Source: CAD feature listing. Evaluate the final solid. Frame: model axes, mm. A direction names the side the tool comes from. Give positions to 0.01 mm unless a question says otherwise; leave off trailing zeros. Loops run counter-clockwise (first coordinate to the right, second up) from the corner with the lowest first, then second, coordinate; pieces in that order, holes last.
from build123d import *

# Parameters (mm, degrees)
SKETCH2_R           = 3.25
SKETCH2_R_2         = 5.25
SKETCH2_R_3         = 2.5
BOSS_EXTRUDE1_DEPTH = 2.5


with BuildPart() as part:
    # Sketch2 → Boss-Extrude1 (new, symmetric)
    with BuildSketch(Plane.XY):
        with BuildLine():
            Line((0, 40), (0, 10))
            ThreePointArc((0, 10), (8.556304179, 0.104761631), (19.583148475, 7.142857143))
            ThreePointArc((19.583148475, 7.142857143), (21.025950646, 9.207134903), (23.416407865, 10))
            Line((23.416407865, 10), (66.583592135, 10))
            ThreePointArc((66.583592135, 10), (68.974049354, 9.207134903), (70.416851525, 7.142857143))
            ThreePointArc((70.416851525, 7.142857143), (81.443695821, 0.104761631), (90, 10))
            Line((90, 10), (90, 20))
            ThreePointArc((90, 20), (88.828427125, 22.828427125), (86, 24))
            Line((86, 24), (70, 24))
            ThreePointArc((70, 24), (50.388386486, 28.00668945), (33.919878771, 39.384615385))
            ThreePointArc((33.919878771, 39.384615385), (33.261138462, 39.839732422), (32.476673921, 40))
            Line((32.476673921, 40), (23.416407865, 40))
            ThreePointArc((23.416407865, 40), (21.025950646, 40.792865097), (19.583148475, 42.857142857))
            ThreePointArc((19.583148475, 42.857142857), (8.556304179, 49.895238369), (0, 40))
        make_face()
        with Locations((10, 40)):
            Circle(SKETCH2_R, mode=Mode.SUBTRACT)
        with Locations((10, 10)):
            Circle(SKETCH2_R_2, mode=Mode.SUBTRACT)
        with Locations((80, 10)):
            Circle(SKETCH2_R_2, mode=Mode.SUBTRACT)
        with Locations((35, 24)):
            Circle(SKETCH2_R_3, mode=Mode.SUBTRACT)
    extrude(amount=BOSS_EXTRUDE1_DEPTH, both=True)


solid = part.part
1) Cut plane A-A (x = 10). Return loops of the section in (y, z).
Checks:
outline: (0, -2.5) - (4.75, -2.5) - (4.75, 2.5) - (0, 2.5) - close; (15.25, -2.5) - (36.75, -2.5) - (36.75, 2.5) - (15.25, 2.5) - close; (43.25, -2.5) - (50, -2.5) - (50, 2.5) - (43.25, 2.5) - close
2) Cut plane C-C (x = 80). Return loops of the section in (y, z), and give its area (3 significant figures).
Checks:
outline: (0, -2.5) - (4.75, -2.5) - (4.75, 2.5) - (0, 2.5) - close; (15.25, -2.5) - (24, -2.5) - (24, 2.5) - (15.25, 2.5) - close
area: 67.5 mm2
3) Reachability of faces 1 (the flat face through (28, 40, 0)), 2 (the cylindrical face through (9.295, 36.827, -0.035)), 3 (the cylindrical face through (21, 9.19, 0.04)) from +Z, -Z, +X, -X, +Y, -Y: full face, straight path, thin tool, end or side. Return the list, or none.
Checks:
face 1: +Z, -Z, +X, +Y
face 2: +Z, -Z
face 3: +Z, -Z, -Y
4) Contact query for flat-ended pins moving along their axis: P1, Ø3, axis at x = 35, y = 24, coming from the -Z side; P2, Ø1.5, axis at x = 77, z = -0.5, coming from the +Y side; P3, Ø3, axis at x = 20.5, z = -1, coming from the -Y side; P4, Ø1.5, axis at x = 43, z = -0.5, coming from the -Y side. Output: stop coordinate, or through.
Checks:
P1: passes through
P2: stops at y = 24
P3: stops at y = 5.64
P4: stops at y = 10
5) Pull-direction query (Y, two-part tool) for faces 4 (the flat face through (78, 24, 0)), 5 (the cylindrical face through (68.945, 9.228, 0.035)), 6 (the cylindrical face through (36.34, 26.11, -0.04)), 7 (the cylindrical face through (12.82, 14.43, -0.04)); classes: released by +Y, released by -Y, zero draft, split by the parting line, or undercut.
Checks:
face 4: released by +Y
face 5: released by -Y
face 6: undercut
face 7: undercut
6) Ray query, probe 1 along Y at (x, z) = (10, -0.15); probe 2 along Y at (x, z) = (7, 1.1); probe 3 along Y at (x, z) = (30, -0.4). Return the intervals inside material, ascending.
Checks:
probe 1: y = 0 to 4.75, 15.25 to 36.75, 43.25 to 50
probe 2: y = 0.46 to 5.69, 14.31 to 38.75, 41.25 to 49.54
probe 3: y = 10 to 40
7) Cut plane B-B (z = -1.15). Return loops of the section in (x, y), and give its area (3 significant figures).
Checks:
outline: (0, 10) arc R10 ccw to (19.58, 7.14) arc R4 cw to (23.42, 10) - (66.58, 10) arc R4 cw to (70.42, 7.14) arc R10 ccw to (90, 10) - (90, 20) arc R4 ccw to (86, 24) - (70, 24) arc R50 cw to (33.92, 39.38) arc R2 ccw to (32.48, 40) - (23.42, 40) arc R4 cw to (19.58, 42.86) arc R10 ccw to (0, 40) - close; hole circle Ø10.5 at (10, 10); hole circle Ø6.5 at (10, 40); hole circle Ø5 at (35, 24); hole circle Ø10.5 at (80, 10)
area: 2,220 mm2
8) Cut plane D-D (y = 11). Return loops of the section in (x, z).
Checks:
outline: (0, -2.5) - (4.85, -2.5) - (4.85, 2.5) - (0, 2.5) - close; (15.15, -2.5) - (74.85, -2.5) - (74.85, 2.5) - (15.15, 2.5) - close; (85.15, -2.5) - (90, -2.5) - (90, 2.5) - (85.15, 2.5) - close
